from build123d import *

# Parameters (mm, degrees)
SKETCH2_W            = 55.515999966
SKETCH2_H            = 31.75
BOSS_EXTRUDE1_DEPTH  = 2.54
SKETCH4_W            = 6.35
SKETCH4_H            = 2.54
BOSS_EXTRUDE7_DEPTH  = 22.86
SKETCH29_W           = 55.515999966
SKETCH29_H           = 2.54
BOSS_EXTRUDE12_DEPTH = 5.08
SKETCH31_W           = 3.81
SKETCH31_H           = 8.89
BOSS_EXTRUDE13_DEPTH = 22.86
SKETCH32_W           = 7
SKETCH32_H           = 25.908
BOSS_EXTRUDE14_DEPTH = 31.75
SKETCH33_R           = 1.65
CUT_EXTRUDE5_DEPTH   = 9.144
SKETCH36_R           = 1.75
CUT_EXTRUDE7_DEPTH   = 2.54
SKETCH37_W           = 42.8
SKETCH37_H           = 2.54
BOSS_EXTRUDE15_DEPTH = 12.7
SKETCH38_W           = 55.5
SKETCH38_H           = 2.54
BOSS_EXTRUDE16_DEPTH = 6.35
CUT_EXTRUDE19_DEPTH  = 17.78
FILLET9_R            = 2.54
FILLET11_R           = 2.54
FILLET12_R           = 2.54
FILLET13_R           = 2.54
SKETCH47_R           = 11
CUT_EXTRUDE21_DEPTH  = 7.112
FILLET17_R           = 1.27
FILLET18_R           = 1.27
FILLET19_R           = 2.54
CUT_EXTRUDE24_DEPTH  = 7.62
SKETCH52_W           = 0.667345496
SKETCH52_H           = 9.289885036
CUT_EXTRUDE25_DEPTH  = 7.62


with BuildPart() as part:
    # Sketch2 → Boss-Extrude1 (new body)
    with BuildSketch(Plane(origin=(0, 0, 0), x_dir=(1, 0, 0), z_dir=(0, 1, 0))):
        with Locations((-1401.125525756, 387.055412371)):
            Rectangle(SKETCH2_W, SKETCH2_H)
    extrude(amount=BOSS_EXTRUDE1_DEPTH)

    # Sketch4 → Boss-Extrude7 (add)
    with BuildSketch(Plane.XZ):
        with Locations((-1376.542525773, -404.200412371)):
            Rectangle(SKETCH4_W, SKETCH4_H)
        with Locations((-1425.692525773, -404.200412371)):
            Rectangle(SKETCH4_W, SKETCH4_H)
    extrude(amount=-BOSS_EXTRUDE7_DEPTH)

    # Sketch29 → Boss-Extrude12 (add)
    with BuildSketch(Plane.XY.offset(-371.180412371)):
        with Locations((-1401.125525756, 1.27)):
            Rectangle(SKETCH29_W, SKETCH29_H)
    extrude(amount=BOSS_EXTRUDE12_DEPTH)

    # Sketch31 → Boss-Extrude13 (add)
    with BuildSketch(Plane.XZ):
        Polygon((-1428.883525739, -366.100412371), (-1373.367525773, -366.100412371), (-1373.367525773, -362.290412371), (-1427.977525773, -362.290412371), (-1431.787525773, -362.290412371), (-1431.787525773, -366.100412371), align=None)
        with Locations((-1429.882525773, -357.845412371)):
            Rectangle(SKETCH31_W, SKETCH31_H)
        Polygon((-1431.787525773, -353.400412371), (-1427.977525773, -353.400412371), (-1427.977525773, -349.590412371), (-1435.597525773, -349.590412371), (-1435.597525773, -353.400412371), align=None)
    extrude(amount=-BOSS_EXTRUDE13_DEPTH)

    # Sketch32 → Boss-Extrude14 (add)
    with BuildSketch(Plane.ZY.offset(1435.597525773)):
        with Locations((-351.526012371, 16.764)):
            Rectangle(SKETCH32_W, SKETCH32_H)
    extrude(amount=BOSS_EXTRUDE14_DEPTH)

    # Sketch33 → Cut-Extrude5 (cut)
    with BuildSketch(Plane.XY.offset(-362.290412371)):
        with Locations((-1402.577525773, 11.43)):
            Circle(SKETCH33_R)
    extrude(amount=-CUT_EXTRUDE5_DEPTH, mode=Mode.SUBTRACT)

    # Sketch36 → Cut-Extrude7 (cut)
    with BuildSketch(Plane(origin=(0, 0, -405.470412371), x_dir=(-1, 0, 0), z_dir=(0, 0, -1))):
        with Locations((1425.117525773, 17.78)):
            Circle(SKETCH36_R)
        with Locations((1425.117525773, 7.78)):
            Circle(SKETCH36_R)
        with Locations((1377.117525773, 17.78)):
            Circle(SKETCH36_R)
        with Locations((1377.117525773, 7.78)):
            Circle(SKETCH36_R)
    extrude(amount=-CUT_EXTRUDE7_DEPTH, mode=Mode.SUBTRACT)

    # Sketch37 → Boss-Extrude15 (add)
    with BuildSketch(Plane(origin=(0, 0, -402.930412371), x_dir=(-1, 0, 0), z_dir=(0, 0, -1))):
        with Locations((1401.117525773, 1.27)):
            Rectangle(SKETCH37_W, SKETCH37_H)
    extrude(amount=BOSS_EXTRUDE15_DEPTH)

    # Sketch38 → Boss-Extrude16 (add)
    with BuildSketch(Plane(origin=(0, 0, -405.470412371), x_dir=(-1, 0, 0), z_dir=(0, 0, -1))):
        with Locations((1401.117525773, 1.27)):
            Rectangle(SKETCH38_W, SKETCH38_H)
    extrude(amount=BOSS_EXTRUDE16_DEPTH)

    # Sketch46 → Cut-Extrude19 (cut)
    with BuildSketch(Plane(origin=(0, 2.54, 0), x_dir=(1, 0, 0), z_dir=(0, 1, 0))):
        with BuildLine():
            Line((-1422.517525773, 415.630412371), (-1428.867525773, 415.630412371))
            Line((-1428.867525773, 415.630412371), (-1428.867525773, 405.470412371))
            ThreePointArc((-1428.867525773, 405.470412371), (-1423.588320876, 409.235284311), (-1422.517525773, 415.630412371))
        make_face()
        with BuildLine():
            Line((-1417.437071461, 366.100412371), (-1428.883525739, 366.100412371))
            Line((-1428.883525739, 366.100412371), (-1428.883525739, 402.930412371))
            ThreePointArc((-1428.883525739, 402.930412371), (-1420.659545742, 397.92062476), (-1417.437071461, 388.846073619))
            Line((-1417.437071461, 388.846073619), (-1417.437071461, 366.100412371))
        make_face()
        with BuildLine():
            Line((-1373.367525773, 405.470412371), (-1373.367525773, 415.630412371))
            Line((-1373.367525773, 415.630412371), (-1379.717525773, 415.630412371))
            ThreePointArc((-1379.717525773, 415.630412371), (-1379.413786034, 408.755874708), (-1373.367525773, 405.470412371))
        make_face()
    extrude(amount=-CUT_EXTRUDE19_DEPTH, mode=Mode.SUBTRACT)

    # Fillet9
    fillet9_edges = [part.edges().sort_by_distance(p)[0] for p in [
        (-1417.437071461, 1.27, -366.100412371),
    ]]
    fillet(fillet9_edges, radius=FILLET9_R)

    # Fillet11
    fillet11_edges = [part.edges().sort_by_distance(p)[0] for p in [
        (-1431.787525773, 11.43, -353.400412371),
    ]]
    fillet(fillet11_edges, radius=FILLET11_R)

    # Fillet12
    fillet12_edges = [part.edges().sort_by_distance(p)[0] for p in [
        (-1427.977525773, 11.43, -362.290412371),
    ]]
    fillet(fillet12_edges, radius=FILLET12_R)

    # Fillet13
    fillet13_edges = [part.edges().sort_by_distance(p)[0] for p in [
        (-1431.787525773, 11.43, -366.100412371),
        (-1427.977525773, 11.43, -349.590412371),
    ]]
    fillet(fillet13_edges, radius=FILLET13_R)

    # Sketch47 → Cut-Extrude21 (cut)
    with BuildSketch(Plane.XY.offset(-348.026012371)):
        with Locations((-1452.107525773, 16.51)):
            Circle(SKETCH47_R)
    extrude(amount=-CUT_EXTRUDE21_DEPTH, mode=Mode.SUBTRACT)

    # Fillet17
    fillet17_edges = [part.edges().sort_by_distance(p)[0] for p in [
        (-1435.597525773, 3.81, -351.495412371),
        (-1435.597525773, 0, -351.495412371),
    ]]
    fillet(fillet17_edges, radius=FILLET17_R)

    # Fillet18
    fillet18_edges = [part.edges().sort_by_distance(p)[0] for p in [
        (-1435.597525773, 13.335, -353.400412371),
        (-1435.597525773, 13.335, -349.590412371),
    ]]
    fillet(fillet18_edges, radius=FILLET18_R - 0.0001)  # a hair under: the kernel refuses the full size

    # Fillet19
    fillet19_edges = [part.edges().sort_by_distance(p)[0] for p in [
        (-1435.597525773, 29.718, -351.526012371),
        (-1435.597525773, 22.86, -351.495412371),
    ]]
    fillet(fillet19_edges, radius=FILLET19_R)

    # Sketch51 → Cut-Extrude24 (cut)
    with BuildSketch(Plane.XY.offset(-348.026012371)):
        with BuildLine():
            Line((-1467.347525773, 29.718), (-1467.347525773, 19.304))
            ThreePointArc((-1467.347525773, 19.304), (-1463.253192632, 26.289780699), (-1455.917525773, 29.718))
            Line((-1455.917525773, 29.718), (-1467.347525773, 29.718))
        make_face()
        with BuildLine():
            ThreePointArc((-1455.917525773, 3.81), (-1463.26939399, 7.220437323), (-1467.347525773, 14.224))
            Line((-1467.347525773, 14.224), (-1467.347525773, 3.81))
            Line((-1467.347525773, 3.81), (-1455.917525773, 3.81))
        make_face()
    extrude(amount=-CUT_EXTRUDE24_DEPTH, mode=Mode.SUBTRACT)

    # Sketch52 → Cut-Extrude25 (cut)
    with BuildSketch(Plane.XY.offset(-348.026012371)):
        with Locations((-1467.013853025, 16.749471922)):
            Rectangle(SKETCH52_W, SKETCH52_H)
    extrude(amount=-CUT_EXTRUDE25_DEPTH, mode=Mode.SUBTRACT)


solid = part.part
Geometry check sheet. Reference: the model listing, model coordinates, mm. A direction names the side the tool comes from. Coordinates: 2 decimals unless noted, no trailing zeros. Order: outer loops, then holes, each group sorted by start corner. A loop starts at its lowest first (then second) coordinate and runs counter-clockwise, first axis right, second up. Notation, with made-up numbers: (-8.5, 13) -> (-1.5, 13) arc R7 ccw to (-1.5, 19) -> close; hole circle Ø6 at (57.5, -8). An arc over 180 degrees is marked (long way). Use a Markdown table: item, result. Add a question column.
1. Set-up check for faces 1 (the face through (-1375.37, 17.86, -404.22)), 2 (the face through (-1431.788, 11, -360)), 3 (the face through (-1417.437, 1, -379)), 4 (the face through (-1427.978, 11, -356)): record each of +Z, -Z, +X, -X, +Y, -Y from which the full face is reachable in a straight line by a thin tool's end or side.
2. Cross-section at C-C (z = -373.5). Enter the section's corners in (x, y), and give its area (3 significant figures).
3. Cross-section at B-B (x = -1407.5). Enter the section's corners in (y, z).
4. Cross-section at D-D (y = 17.78). Give the number of separate pieces and of enclosed holes in the cut face, and give its area (3 significant figures).
5. Mould release check, pull along X, two halves, no side actions. Record for faces 5 (the face through (-1462.491, 26.935, -351.477)), 6 (the face through (-1422.518, 13, -404)), 7 (the face through (-1377, 13, -402.93)): pulls with the +X half, pulls with the -X half, needs draft (parallel to the pull), parting line crosses it, or undercut.
6. Go/stop test with flat-tipped pins: pin 1 Ø1 at (x, y) = (-1429.5, 15.5) entering from -Z; pin 2 Ø7.5 at (y, z) = (18, -352) entering from +X; pin 3 Ø3 at (x, y) = (-1425.12, 17.78) entering from +Z; pin 4 Ø2 at (x, z) = (-1394.5, -379) entering from -Y. Record where each tip stops, or that it passes through.
7. Material ranges on L1, parallel to Z at x = -1392, y = 11.75; L2, parallel to Y at x = -1394, z = -387.5; L3, parallel to Z at x = -1444.5, y = 27.75, recorded low to high.
8. Cross-section at A-A (x = -1457). Enter the section's corners in (y, z), and give its area (3 significant figures).
Filled sheet:
| question | item | result |
|---|---|---|
| 1 | face 1 | -Z |
| 1 | face 2 | -Z, -X, +Y, -Y |
| 1 | face 3 | -X, +Y, -Y |
| 1 | face 4 | +Z, +X, +Y, -Y |
| 2 | outline | (-1417.44, 0) -> (-1373.37, 0) -> (-1373.37, 2.54) -> (-1417.44, 2.54) -> close |
| 2 | area | 112 mm2 |
| 3 | outline | (0, -415.63) -> (2.54, -415.63) -> (2.54, -366.1) -> (22.86, -366.1) -> (22.86, -362.29) -> (0, -362.29) -> close |
| 4 | separate pieces | 6 |
| 4 | enclosed holes | 0 |
| 4 | area | 365 mm2 |
| 5 | face 5 | pulls with the -X half |
| 5 | face 6 | undercut |
| 5 | face 7 | needs draft |
| 6 | pin 1 | z = -366.1 |
| 6 | pin 2 | x = -1427.98 |
| 6 | pin 3 | z = -362 |
| 6 | pin 4 | y = 0 |
| 7 | L1 | -366.1 to -362.29 |
| 7 | L2 | 0 to 2.54 |
| 7 | L3 | -355.03 to -348.03 |
| 8 | outline | (4, -355.03) -> (6.66, -355.03) -> (6.66, -348.03) -> (4, -348.03) -> close; (26.36, -355.03) -> (29.53, -355.03) -> (29.53, -348.03) -> (26.36, -348.03) -> close |
| 8 | area | 40.8 mm2 |
